```python
from build123d import *

# Parameters (mm, degrees)
ESQUISSE1_R        = 6
BOSS_EXTRU_1_DEPTH = 80
CONG_1_R           = 2


with BuildPart() as part:
    # Esquisse1 → Boss.-Extru.1 (new body)
    with BuildSketch(Plane.XY):
        Circle(ESQUISSE1_R)
    extrude(amount=BOSS_EXTRU_1_DEPTH)

    # Esquisse4 → Révolution1 (revolve)
    with BuildSketch(Plane(origin=(0, 0, 0), x_dir=(1, 0, 0), z_dir=(0, 1, 0))):
        Polygon((0, 0), (0, 12), (-6, 0), align=None)
    revolve(axis=Axis((0, 0, 0), (0, 0, -1)))

    # Congé1
    cong_1_edges = [part.edges().sort_by_distance(p)[0] for p in [
        (-6, 0, 80),
    ]]
    fillet(cong_1_edges, radius=CONG_1_R)


solid = part.part
```
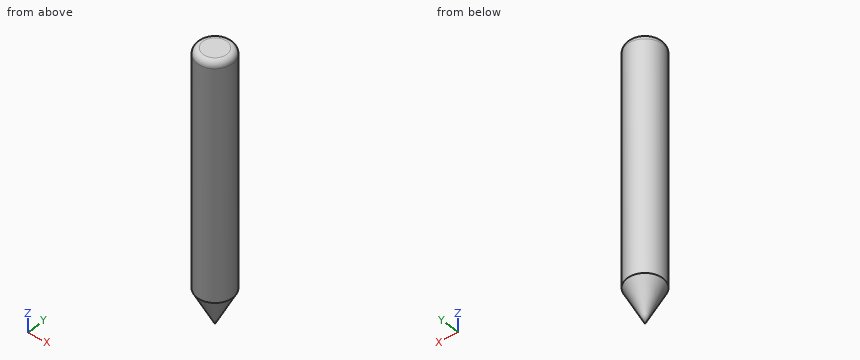
Work out the finished part from the listing and answer in its coordinate system (mm). Coordinates: 2 decimals unless noted, no trailing zeros. Loops run counter-clockwise (first coordinate to the right, second up) from the corner with the lowest first, then second, coordinate; pieces in that order, holes last.
1) Flat-ended cylindrical pins translate along their axes: pin 1 (2 mm diameter, centred on x = 4, z = 11.5, fed in from +Y); pin 2 (2 mm diameter, centred on x = 1.5, z = 18.5, fed in from -Y); pin 3 (2 mm diameter, centred on x = -0.5, y = 3, fed in from -Z); pin 4 (1.5 mm diameter, centred on y = -0.5, z = 57.5, fed in from +X). Find the tip coordinate at first contact, or state that the pin passes through.
Results:
pin 1: stops at y = 5.2
pin 2: stops at y = -5.98
pin 3: stops at z = -7.92
pin 4: stops at x = 6
2) Consider probe 1 along X at (y, z) = (-0.25, 16.5); probe 2 along X at (y, z) = (3, 2.5); probe 3 along Z at (x, y) = (2.75, -1). Determine where each line is inside the solid, lowest interval first.
Results:
probe 1: x = -5.99 to 5.99
probe 2: x = -5.2 to 5.2
probe 3: z = -6.15 to 80
3) Section A-A (z = -1) is taken. Give the vertices of the cut face in (x, y).
Results:
outline: circle Ø11 at (0, 0)
4) Section B-B (z = 31) is taken. Give the vertices of the cut face in (x, y).
Results:
outline: circle Ø12 at (0, 0)
